```python
from build123d import *

# Parameters (mm, degrees)
BOSS_EXTRUDE1_DEPTH = 30.48
SKETCH3_R           = 24.13
CUT_EXTRUDE4_DEPTH  = 90.914560616
SKETCH4_R           = 3.175
CUT_EXTRUDE5_DEPTH  = 63.754
CIRPATTERN3_COUNT   = 6
SKETCH6_W           = 3.81
SKETCH6_H           = 10.509433013
CUT_EXTRUDE6_DEPTH  = 6.35
SKETCH7_W           = 3.7592
SKETCH7_H           = 10.16
BOSS_EXTRUDE4_DEPTH = 5.969
SKETCH8_R           = 1.980775352
CUT_EXTRUDE7_DEPTH  = 5.969
SKETCH9_R           = 2.056796453
CUT_EXTRUDE8_DEPTH  = 12.319
FILLET4_R           = 5.08


with BuildPart() as part:
    # Sketch1 → Boss-Extrude1 (new body)
    with BuildSketch(Plane(origin=(0, 0, 0), x_dir=(1, 0, 0), z_dir=(0, 1, 0))):
        with BuildLine():
            Line((-78.958715675, 0), (-17.998715675, 0))
            ThreePointArc((-17.998715675, 0), (-48.478715675, 30.349942827), (-78.958715675, 0))
        make_face()
    extrude(amount=BOSS_EXTRUDE1_DEPTH)

    # Sketch3 → Cut-Extrude4 (cut, through all)
    with BuildSketch(Plane(origin=(0, 0, 0), x_dir=(1, 0, 0), z_dir=(0, 1, 0))):
        with Locations((-48.478715675, 0)):
            Circle(SKETCH3_R)
    extrude(amount=CUT_EXTRUDE4_DEPTH, mode=Mode.SUBTRACT)

    # Sketch4 → Cut-Extrude5 (cut)
    with BuildSketch(Plane.XY):
        with Locations((-48.824364134, 15.798935299)):
            Circle(SKETCH4_R)
    cut_extrude5 = extrude(amount=-CUT_EXTRUDE5_DEPTH, mode=Mode.SUBTRACT)

    # CirPattern3: Cut-Extrude5 ×6 about axis
    cirpattern3_axis = Axis((-48.478715675, 30.48, 0.130335837), (0, -1, 0))
    for i in range(1, CIRPATTERN3_COUNT):
        add(cut_extrude5.rotate(cirpattern3_axis, i * 360 / CIRPATTERN3_COUNT), mode=Mode.SUBTRACT)

    # Sketch6 → Cut-Extrude6 (cut)
    with BuildSketch(Plane.XY):
        with Locations((-21.173715675, 15.414716507)):
            Rectangle(SKETCH6_W, SKETCH6_H)
    extrude(amount=-CUT_EXTRUDE6_DEPTH, mode=Mode.SUBTRACT)

    # Sketch7 → Boss-Extrude4 (add)
    with BuildSketch(Plane.XY):
        with Locations((-75.783715675, 15.494)):
            Rectangle(SKETCH7_W, SKETCH7_H)
    extrude(amount=BOSS_EXTRUDE4_DEPTH)

    # Sketch8 → Cut-Extrude7 (cut)
    with BuildSketch(Plane(origin=(-73.904115675, 0, 0), x_dir=(0, 0, -1), z_dir=(1, 0, 0))):
        with Locations((-3.048, 15.494)):
            Circle(SKETCH8_R)
    extrude(amount=-CUT_EXTRUDE7_DEPTH, mode=Mode.SUBTRACT)

    # Sketch9 → Cut-Extrude8 (cut)
    with BuildSketch(Plane(origin=(-23.078715675, 0, 0), x_dir=(0, 0, -1), z_dir=(1, 0, 0))):
        with Locations(Location((3.048, 15.24, 0), (0, 0, 180))):
            Circle(SKETCH9_R)
    extrude(amount=CUT_EXTRUDE8_DEPTH, mode=Mode.SUBTRACT)

    # Fillet4
    fillet4_edges = [part.edges().sort_by_distance(p)[0] for p in [
        (-48.478715675, 30.48, -24.13),
    ]]
    fillet(fillet4_edges, radius=FILLET4_R)


solid = part.part
```
For this review, take the finished solid that the model builds, in its own axes (mm). A direction names the side the tool comes from. Round coordinates to 2 decimals unless told otherwise and drop trailing zeros. Order: outer loops, then holes, each group sorted by start corner. A loop starts at its lowest first (then second) coordinate and runs counter-clockwise, first axis right, second up. Notation, with made-up numbers: (-38, 68) -> (3, 68) arc R7 cw to (3, 76) -> close; hole circle Ø2 at (57.5, 4). An arc over 180 degrees is marked (long way). Use a Markdown table: item, result.
Item 1: For line 1 along X through (y, z) = (16, -11.5); line 2 along X through (y, z) = (6.5, -1); line 3 along X through (y, z) = (17.5, 2.5), list the stretches that pass through material, from the lowest coordinate up. Write a range as [from, to].
Resolved:
| item | result |
|---|---|
| line 1 | x = [-76.65, -75.65], [-22.69, -20.3] |
| line 2 | x = [-78.94, -72.59], [-24.37, -18.02] |
| line 3 | x = [-77.66, -73.9] |
Item 2: For pin 1 (1.1 mm diameter, centred on x = -20.5, y = 18, fed in from +Z); pin 2 (1.1 mm diameter, centred on x = -76, z = 3.5, fed in from -Y); pin 3 (3 mm diameter, centred on y = 13.5, z = 3, fed in from +X), all flat-tipped, find the tip position at first contact; note any pin that passes through.
Resolved:
| item | result |
|---|---|
| pin 1 | stops at z = -6.35 |
| pin 2 | stops at y = 10.41 |
| pin 3 | stops at x = -73.9 |
Item 3: Draft analysis for pull direction X (two halves, no side actions). For faces 4 (the cylindrical face through (-47.81, 11.64, -30.343)), 5 (the flat face through (-78, 15, 0)), 6 (the flat face through (-77.663, 13, 3)), 7 (the cylindrical face through (-45.891, 14.583, -27.062)), state which applies: +X half, -X half, draft (parallel to the pull), parting line (faces both ways), or undercut.
Resolved:
| item | result |
|---|---|
| face 4 | parting line |
| face 5 | draft |
| face 6 | -X half |
| face 7 | undercut |
Item 4: Machinability: for faces 1 (the flat face through (-19.269, 13, -3)), 2 (the flat face through (-73.904, 13, 3)), 3 (the flat face through (-76, 10.414, 3)), which of the approach directions +Z, -Z, +X, -X, +Y, -Y give a long, thin tool a straight path to every point of the face, cutting with its end or side? Answer none if there is none.
Resolved:
| item | result |
|---|---|
| face 1 | +Z |
| face 2 | +Z, +X, +Y, -Y |
| face 3 | +Z, +X, -X, -Y |
Item 5: Take a section at A-A (z = 4). State the section outline as (x, y) points.
Resolved:
| item | result |
|---|---|
| outline | (-77.66, 10.41) -> (-73.9, 10.41) -> (-73.9, 13.76) -> (-77.66, 13.76) -> close; (-77.66, 17.23) -> (-73.9, 17.23) -> (-73.9, 20.57) -> (-77.66, 20.57) -> close |
